```python
from build123d import *

# Parameters (mm, degrees)
EXTRUDE_3_DEPTH     = 3
SKETCH_1_4_W        = 10
SKETCH_1_4_H        = 10
EXTRUDE_4_DEPTH     = 33
SKETCH_3_R          = 1.45
CUT_EXTRUDE_1_DEPTH = 16
SKETCH_4_R          = 1.45
CUT_EXTRUDE_2_DEPTH = 16
SKETCH_5_R          = 1.45
CUT_EXTRUDE_3_DEPTH = 16
SKETCH_5_3_R        = 1.45
CUT_EXTRUDE_4_DEPTH = 16
SKETCH_7_W          = 80
SKETCH_7_H          = 4
SKETCH_7_W_2        = 4
SKETCH_7_H_2        = 80
EXTRUDE_5_DEPTH     = 16
CUT_EXTRUDE_5_DEPTH = 16
CUT_EXTRUDE_6_DEPTH = 16
CUT_EXTRUDE_7_DEPTH = 16
CUT_EXTRUDE_8_DEPTH = 16


with BuildPart() as part:
    # Sketch 1 → Extrude 3 (new body)
    with BuildSketch(Plane.XY):
        Polygon((10, 10), (10, 0), (90, 0), (90, 10), (100, 10), (100, 90), (90, 90), (90, 100), (10, 100), (10, 90), (0, 90), (0, 10), align=None)
    extrude(amount=EXTRUDE_3_DEPTH)

    # Sketch 1_4 → Extrude 4 (add)
    with BuildSketch(Plane.XY):
        with Locations((5, 5)):
            Rectangle(SKETCH_1_4_W, SKETCH_1_4_H)
        with Locations((5, 95)):
            Rectangle(SKETCH_1_4_W, SKETCH_1_4_H)
        with Locations((95, 95)):
            Rectangle(SKETCH_1_4_W, SKETCH_1_4_H)
        with Locations((95, 5)):
            Rectangle(SKETCH_1_4_W, SKETCH_1_4_H)
    extrude(amount=EXTRUDE_4_DEPTH)

    # Sketch 3 → Cut-Extrude 1 (cut)
    with BuildSketch(Plane.XY.offset(33)):
        with Locations((5, 95)):
            Circle(SKETCH_3_R)
    extrude(amount=-CUT_EXTRUDE_1_DEPTH, mode=Mode.SUBTRACT)

    # Sketch 4 → Cut-Extrude 2 (cut)
    with BuildSketch(Plane.XY.offset(33)):
        with Locations((95, 95)):
            Circle(SKETCH_4_R)
    extrude(amount=-CUT_EXTRUDE_2_DEPTH, mode=Mode.SUBTRACT)

    # Sketch 5 → Cut-Extrude 3 (cut)
    with BuildSketch(Plane.XY.offset(33)):
        with Locations((5, 5)):
            Circle(SKETCH_5_R)
    extrude(amount=-CUT_EXTRUDE_3_DEPTH, mode=Mode.SUBTRACT)

    # Sketch 5_3 → Cut-Extrude 4 (cut)
    with BuildSketch(Plane.XY.offset(33)):
        with Locations((95, 5)):
            Circle(SKETCH_5_3_R)
    extrude(amount=-CUT_EXTRUDE_4_DEPTH, mode=Mode.SUBTRACT)

    # Sketch 7 → Extrude 5 (add)
    with BuildSketch(Plane.XY.offset(3)):
        Polygon((93, 10), (95, 10), (97, 10), (97, 90), (93, 90), align=None)
        with Locations((50, 5)):
            Rectangle(SKETCH_7_W, SKETCH_7_H)
        with Locations((5, 50)):
            Rectangle(SKETCH_7_W_2, SKETCH_7_H_2)
        with Locations((50, 95)):
            Rectangle(SKETCH_7_W, SKETCH_7_H)
    extrude(amount=EXTRUDE_5_DEPTH)

    # Sketch 8 → Cut-Extrude 5 (cut)
    with BuildSketch(Plane(origin=(0, 7, 0), x_dir=(1, 0, 0), z_dir=(0, 1, 0))):
        Polygon((89.910217028, -19), (50, -3), (10, -19), align=None)
    extrude(amount=-CUT_EXTRUDE_5_DEPTH, mode=Mode.SUBTRACT)

    # Sketch 9 → Cut-Extrude 6 (cut)
    with BuildSketch(Plane(origin=(7, 0, 0), x_dir=(0, 0, -1), z_dir=(1, 0, 0))):
        Polygon((-19, 10), (-3, 50), (-19, 90), align=None)
    extrude(amount=-CUT_EXTRUDE_6_DEPTH, mode=Mode.SUBTRACT)

    # Sketch 10 → Cut-Extrude 7 (cut)
    with BuildSketch(Plane.XZ.offset(-93)):
        Polygon((10, 19), (50, 3), (90, 19), align=None)
    extrude(amount=-CUT_EXTRUDE_7_DEPTH, mode=Mode.SUBTRACT)

    # Sketch 11 → Cut-Extrude 8 (cut)
    with BuildSketch(Plane.ZY.offset(-93)):
        Polygon((19, 90), (3, 50), (19, 10), align=None)
    extrude(amount=-CUT_EXTRUDE_8_DEPTH, mode=Mode.SUBTRACT)


solid = part.part
```
Input: part model. Units: mm. Frame: model coordinates. A direction names the side the tool comes from. Round coordinates to 2 decimals unless told otherwise and drop trailing zeros. Write each loop counter-clockwise with the first axis right and the second up, starting at its lowest first coordinate (ties: lowest second). Pieces come first, ordered by that corner, then holes. Notation, with made-up numbers: (49.5, -32) -> (69.5, -32) arc R29 ccw to (69.5, -10) -> close; hole circle Ø10 at (9.25, 64). An arc over 180 degrees is marked (long way). Answer as CSV lines item,"result".
1. Reachability of faces 4 (the flat face through (79, 97, 7)), 5 (the flat face through (5, 70, 11)), 6 (the flat face through (49, 2, 3)), 7 (the flat face through (90, 95, 21)) from +Z, -Z, +X, -X, +Y, -Y: full face, straight path, thin tool, end or side. Return the list, or none.
Geometry says:
face 4,"+Z, +Y"
face 5,"+Z, +X, -X"
face 6,"+Z, -Y"
face 7,"+Z"
2. Section D-D (y = 95). Return the cut outline in (x, z), plus the area to 3 significant figures.
Geometry says:
outline,"(0, 0) -> (100, 0) -> (100, 33) -> (96.45, 33) -> (96.45, 17) -> (93.55, 17) -> (93.55, 33) -> (90, 33) -> (90, 19) -> (50, 3) -> (10, 19) -> (10, 33) -> (6.45, 33) -> (6.45, 17) -> (3.55, 17) -> (3.55, 33) -> (0, 33) -> close"
area,"1,450 mm^2"
3. Section C-C (y = 5). Return the cut outline in (x, z), plus the area to 3 significant figures.
Geometry says:
outline,"(0, 0) -> (100, 0) -> (100, 33) -> (96.45, 33) -> (96.45, 17) -> (93.55, 17) -> (93.55, 33) -> (90, 33) -> (90, 19) -> (89.91, 19) -> (50, 3) -> (10, 19) -> (10, 33) -> (6.45, 33) -> (6.45, 17) -> (3.55, 17) -> (3.55, 33) -> (0, 33) -> close"
area,"1,450 mm^2"
4. Mould query, pull axis X, two halves, no side actions, for faces 1 (the flat face through (97, 25, 9)), 2 (the flat face through (93, 75, 9)), 3 (the flat face through (3.8, 6.2, 33)). Classes: +X half, -X half, draft (parallel to the pull), parting line (faces both ways), or undercut.
Geometry says:
face 1,"+X half"
face 2,"undercut"
face 3,"draft"
5. Ray query, L1, parallel to X at y = 95, z = 23; L2, parallel to Y at x = 88, z = 15. Return the intervals inside material, ascending. Write a range as [from, to].
Geometry says:
L1,"x = [0, 3.55], [6.45, 10], [90, 93.55], [96.45, 100]"
L2,"y = [3, 7], [93, 97]"
6. Section A-A (z = 21). Return the cut outline in (x, y), plus the area to 3 significant figures.
Geometry says:
outline,"(0, 0) -> (10, 0) -> (10, 10) -> (0, 10) -> close; (0, 90) -> (10, 90) -> (10, 100) -> (0, 100) -> close; (90, 0) -> (100, 0) -> (100, 10) -> (90, 10) -> close; (90, 90) -> (100, 90) -> (100, 100) -> (90, 100) -> close; hole circle Ø2.9 at (5, 5); hole circle Ø2.9 at (5, 95); hole circle Ø2.9 at (95, 5); hole circle Ø2.9 at (95, 95)"
area,"374 mm^2"
7. Contact query for flat-ended pins moving along their axis: P1, Ø0.9, axis at x = 5.5, y = 95.5, coming from the +Z side; P2, Ø6, axis at x = 10.5, y = 34, coming from the +Z side; P3, Ø8, axis at y = 83, z = 27, coming from the -X side; P4, Ø12, axis at x = 75.5, z = 18, coming from the +Y side. Output: stop coordinate, or through.
Geometry says:
P1,"stops at z = 17"
P2,"stops at z = 3"
P3,"passes through"
P4,"stops at y = 97"
8. Section B-B (x = 34.5). Return the cut outline in (y, z).
Geometry says:
outline,"(0, 0) -> (100, 0) -> (100, 3) -> (97, 3) -> (97, 9.2) -> (93, 9.2) -> (93, 3) -> (7, 3) -> (7, 9.2) -> (3, 9.2) -> (3, 3) -> (0, 3) -> close"
